Work out the finished part from the listing and answer in its coordinate system (mm). A direction names the side the tool comes from. Give positions to 0.01 mm unless a question says otherwise; leave off trailing zeros. Write item = value, one per line.
from build123d import *

# Parameters (mm, degrees)
F1_DEPTH  = 1
F3_DEPTH  = 11
F4_DEPTH  = 10
F5_W      = 1.2
F5_H      = 0.6395594371
F6_REACH  = 15.595486632
F7_SIZE2  = 0.267939
F7_SIZE   = 0.99999
F8_D      = 2
F8_DEPTH  = 2
F8_TIP    = 0.600860619
F10_D     = 5
F10_DEPTH = 5
F10_TIP   = 1.5021515476
F11_D     = 4
F11_DEPTH = 2
F11_TIP   = 1.2017212381
F14_DEPTH = 1
F16_DEPTH = 1


# Not quite as in the source:
# - a fillet or chamfer is up to 0.001 mm smaller than in the source, because OpenCascade refuses the exact size
# - a feature names something its author has since deleted; it is built from what else it names


with BuildPart() as f1:
    # F0 (on Top) → F1 (new body)
    with BuildSketch(Plane.XY):
        Polygon((-18.5, 4), (-18.5, 0), (-18.5, -4), (-17, -4), (-17, -2.5), (-15, -2.5), (-14, -6), (0, -6), (0, 6), (-10.2, 6), (-10.2, -0.1), (-13.1, -0.1), (-13.1, 3.1), (-14.4, 3.1), (-14.4, 6), (-15, 2.5), (-17, 2.5), (-17, 4), align=None)
        Polygon((-10.2, 6), (-14.4, 6), (-14.4, 3.1), (-13.1, 3.1), (-13.1, -0.1), (-10.2, -0.1), align=None)
        Polygon((-11, 5.2), (-11, 0.7), (-12.3, 0.7), (-12.3, 3.9), (-13.6, 3.9), (-13.6, 5.2), align=None, mode=Mode.SUBTRACT)
        Polygon((-12.3, 0.7), (-11, 0.7), (-11, 5.2), (-13.6, 5.2), (-13.6, 3.9), (-12.3, 3.9), align=None)
    extrude(amount=F1_DEPTH)

    # F2 (on Right) → F3 (join)
    with BuildSketch(Plane.YZ):
        Polygon((-6, 0), (-4.9647238196, 0), (-4.0316277581, 3.4823619098), (-2.9361313709, 7.5708100863), (-3.9020571972, 7.8296291314), align=None)
        Polygon((4.9647238196, 0), (6, 0), (7.2940952255, 4.8296291314), (6.3281693992, 5.0884481765), (5.232673012, 1), align=None)
        Polygon((-4.9647238196, 0), (4.9647238196, 0), (5.232673012, 1), (-4.0316277581, 3.4823619098), align=None)
        Polygon((-4.0316277581, 3.4823619098), (5.232673012, 1), (6.3281693992, 5.0884481765), (-2.9361313709, 7.5708100863), align=None)
    extrude(amount=-F3_DEPTH)

    # F2 (on Right) → F4 (cut)
    with BuildSketch(Plane.YZ):
        Polygon((-4.0316277581, 3.4823619098), (5.232673012, 1), (6.3281693992, 5.0884481765), (-2.9361313709, 7.5708100863), align=None)
    extrude(amount=-F4_DEPTH, mode=Mode.SUBTRACT)

    f6_end = Plane(origin=(-8.4427376171, 0.0169846051, 0), x_dir=(-1, 0, 0), z_dir=(0, 0, -1))
    # F5 (on face) → F6 (join, up to a plane its end follows)
    with BuildSketch(Plane(origin=(0, 1.6960190142, 6.3296291314), x_dir=(1, 0, 0), z_dir=(0, 0.2588190451, 0.9659258263))):
        Polygon((-15.2, 5.7955549577), (-15.2, 2.7955549577), (-14, 2.7955549577), (-14, 2.1559955206), (-14, -0.4044450423), (-11, -0.4044450423), (-11, 5.7955549577), align=None)
        Polygon((-11.9, 4.8955549577), (-11.9, 0.4955549577), (-13.1, 0.4955549577), (-13.1, 3.6955549577), (-14.3, 3.6955549577), (-14.3, 4.8955549577), align=None, mode=Mode.SUBTRACT)
        with Locations((-14.6, 2.4757752392)):
            Rectangle(F5_W, F5_H)
    f6_long = extrude(amount=-F6_REACH, mode=Mode.PRIVATE)
    add(split(f6_long, bisect_by=f6_end, keep=Keep.BOTTOM, mode=Mode.PRIVATE))

    # F7 (size 1 and 0.2679491924 in the source; OpenCascade refuses exactly that, so slightly less here)
    f7_edges = [f1.edges().sort_by_distance(p)[0] for p in [
        (-7, -6, 1),
    ]]
    f7_side = f1.faces().sort_by_distance((-7, -6, 0.5))[0]
    chamfer(f7_edges, length=F7_SIZE, length2=F7_SIZE2, reference=f7_side)

    # F8
    with Locations(Plane(origin=(0, 0, 0), x_dir=(1, 0, 0), z_dir=(0, 0, -1))):
        with Locations((-14, 0)):
            Hole(F8_D / 2, depth=F8_DEPTH)
            with Locations((0, 0, -(F8_DEPTH + F8_TIP / 2))):  # 118° drill point
                Cone(0, F8_D / 2, F8_TIP, mode=Mode.SUBTRACT)

    # F10
    with Locations(Plane(origin=(0, 0, 0), x_dir=(1, 0, 0), z_dir=(0, 0, -1))):
        with Locations((-6.7131645046, 0), (0, 0)):
            Hole(F10_D / 2, depth=F10_DEPTH)
            with Locations((0, 0, -(F10_DEPTH + F10_TIP / 2))):  # 118° drill point
                Cone(0, F10_D / 2, F10_TIP, mode=Mode.SUBTRACT)

    # F11 (one way)
    with BuildSketch(Plane(origin=(0, 0, 1), x_dir=(1, 0, 0), z_dir=(0, 0, -1))):
        with Locations((-14, 0)):
            Circle(F11_D / 2)
    extrude(amount=-F11_DEPTH, mode=Mode.SUBTRACT)
    with Locations(Plane(origin=(0, 0, 1), x_dir=(1, 0, 0), z_dir=(0, 0, -1))):
        with Locations((-14, 0)):
            with Locations((0, 0, -(F11_DEPTH + F11_TIP / 2))):  # 118° drill point
                Cone(0, F11_D / 2, F11_TIP, mode=Mode.SUBTRACT)

    # F12: F1 across plane


with BuildPart() as f1_1:
    add(f1.part)
    add(f1.part.mirror(Plane.YZ))

    # F13 (on face) → F14 (cut)
    with BuildSketch(Plane(origin=(0, -5.5980762114, 1.5), x_dir=(1, 0, 0), z_dir=(0, -0.9659258263, 0.2588190451))):
        with BuildLine():
            Line((0, 6.5529142706), (-2.8882349873, 6.5529142706))
            ThreePointArc((-2.8882349873, 6.5529142706), (0, 5.3202412586), (2.8882349873, 6.5529142706))
            Line((2.8882349873, 6.5529142706), (0, 6.5529142706))
        make_face()
    extrude(amount=-F14_DEPTH, mode=Mode.SUBTRACT)

    # F15 (on face) → F16 (cut, through all)
    with BuildSketch(Plane(origin=(0, 5.5980762114, -1.5), x_dir=(-1, 0, 0), z_dir=(0, 0.9659258263, -0.2588190451))):
        Polygon((-7.5, 6.5529142706), (-10, 6.5529142706), (-10, 2.3202412586), (-6, 2.3202412586), (-6, 4.3202412586), (-7.5, 5.5958246812), align=None)
    extrude(amount=-F16_DEPTH, mode=Mode.SUBTRACT)


solid = f1_1.part
1. Given pin 1 (1 mm diameter, centred on y = 2, z = 3.5, fed in from -X); pin 2 (2.5 mm diameter, centred on x = 14, y = 0, fed in from -Z); pin 3 (2.5 mm diameter, centred on y = 2.5, z = 4, fed in from +X); pin 4 (1.1 mm diameter, centred on x = -18, z = 0.5, fed in from +Y), each flat-ended and moving along its own axis, determine where each tip first touches the part or whether it passes through.
Solution:
pin_1 = -14
pin_2 = 0
pin_3 = 15.2
pin_4 = 4
2. For a pull along X with two mould halves and no side action, classify faces 4 (the flat face through (12.19, 0.75, 4.36)), 5 (the flat face through (11, -2, 4)), 6 (the flat face through (13.1, 3, 3)) as pulls with the +X half, pulls with the -X half, needs draft (parallel to the pull), parting line crosses it, or undercut.
Solution:
face_4 = needs draft
face_5 = pulls with the +X half
face_6 = undercut
3. Straight lines are drawn through the part: line 1 (X direction, y = 1.25, z = 5.75); line 2 (Y direction, x = -14, z = 0.65); line 3 (Y direction, x = 14, z = 0.35). For each, find the intervals that lie inside material, in ascending order.
Solution:
line_1 = -14 to -10, 10 to 14
line_2 = -5.83 to -1, 1 to 6.17
line_3 = -5.91 to -1, 1 to 6.09
4. Find section C-C, the plane z = 4.5. Give the number of separate pieces and of enclosed holes in the cut face, then the cut area to 3 significant figures.
Solution:
separate_pieces = 1
enclosed_holes = 2
area = 96.5 mm^2
5. A tool of negligible diameter and unlimited length cuts with its end or side. For faces 1 (the flat face through (-16, -2.5, 0.5)), 2 (the flat face through (-13.1, 3, 3)), 3 (the flat face through (-17, 3.2, 0.5)), from which of +Z, -Z, +X, -X, +Y, -Y can it reach the whole face along a straight path? Write none if from no direction.
Solution:
face_1 = +Z, -Z, -Y
face_2 = none
face_3 = +Z, -Z, +Y
